```python
from build123d import *

# Parameters (mm, degrees)
MAIN_SIDE_DEPTH          = 3.175
SKETCH2_W                = 12.573
SKETCH2_H                = 3.048
BOTTOM_PLATE_HOLES_DEPTH = 254.555547868
SKETCH3_W                = 12.7
SKETCH3_H                = 3.048
CUT_EXTRUDE1_DEPTH       = 254.555547868
SKETCH4_W                = 3.048
SKETCH4_H                = 12.573
CUT_EXTRUDE2_DEPTH       = 254.555547868
SKETCH5_W                = 3.175
SKETCH5_H                = 31.75
CUT_EXTRUDE3_DEPTH       = 254.555547868
SKETCH6_R                = 9.525
CUT_EXTRUDE4_DEPTH       = 254.555547868
SKETCH7_W                = 12.7
SKETCH7_H                = 3.175
CUT_EXTRUDE5_DEPTH       = 254.555547868
SKETCH8_W                = 3.175
SKETCH8_H                = 12.7
CUT_EXTRUDE6_DEPTH       = 254.555547868
BOSS_EXTRUDE2_DEPTH      = 3.175
SKETCH10_R               = 1.75
SKETCH10_R_2             = 7.62
CUT_EXTRUDE7_DEPTH       = 254.555547868
FILLET1_R                = 6.35
SKETCH14_R               = 3.81
SKETCH14_W               = 3.175
SKETCH14_H               = 6.35
CUT_EXTRUDE8_DEPTH       = 254.555547868
CUT_EXTRUDE9_DEPTH       = 254.555547868
CUT_EXTRUDE10_DEPTH      = 254.555547868
FILLET2_R                = 6.35


with BuildPart() as part:
    # Sketch1 → Main Side (new body)
    with BuildSketch(Plane.XY):
        Polygon((62.123903317, 7.421650144), (131.966346795, 7.421650144), (147.472889282, 13.771650144), (201.808790274, 13.771650144), (201.808790274, 77.271650144), (151.008790274, 77.271650144), (151.008790274, 153.471650144), (86.008898009, 153.471650144), (79.342261849, 77.271650144), (-42.539209726, 77.271650144), (-42.539209726, 13.771650144), (46.617360741, 13.771650144), align=None)
    extrude(amount=MAIN_SIDE_DEPTH)

    # Sketch2 → Bottom Plate Holes (cut, through all)
    with BuildSketch(Plane.XY.offset(3.175)):
        with Locations((141.483790274, 29.265650144)):
            Rectangle(SKETCH2_W, SKETCH2_H)
        with Locations((20.833790274, 29.265650144)):
            Rectangle(SKETCH2_W, SKETCH2_H)
    extrude(amount=-BOTTOM_PLATE_HOLES_DEPTH, mode=Mode.SUBTRACT)

    # Sketch3 → Cut-Extrude1 (cut, through all)
    with BuildSketch(Plane.XY.offset(3.175)):
        with Locations((119.258790274, 70.413650144)):
            Rectangle(SKETCH3_W, SKETCH3_H)
    extrude(amount=-CUT_EXTRUDE1_DEPTH, mode=Mode.SUBTRACT)

    # Sketch4 → Cut-Extrude2 (cut, through all)
    with BuildSketch(Plane.XY.offset(3.175)):
        with Locations((-41.015209726, 45.521650144)):
            Rectangle(SKETCH4_W, SKETCH4_H)
    extrude(amount=-CUT_EXTRUDE2_DEPTH, mode=Mode.SUBTRACT)

    # Sketch5 → Cut-Extrude3 (cut, through all)
    with BuildSketch(Plane.XY.offset(3.175)):
        with Locations((193.871290274, 61.396650144)):
            Rectangle(SKETCH5_W, SKETCH5_H)
    extrude(amount=-CUT_EXTRUDE3_DEPTH, mode=Mode.SUBTRACT)

    # Sketch6 → Cut-Extrude4 (cut, through all)
    with BuildSketch(Plane.XY.offset(3.175)):
        with Locations((-2.114209726, 51.856650144)):
            Circle(SKETCH6_R)
    extrude(amount=-CUT_EXTRUDE4_DEPTH, mode=Mode.SUBTRACT)

    # Sketch7 → Cut-Extrude5 (cut, through all)
    with BuildSketch(Plane.XY.offset(3.175)):
        with Locations((118.508844141, 151.884150144)):
            Rectangle(SKETCH7_W, SKETCH7_H)
    extrude(amount=-CUT_EXTRUDE5_DEPTH, mode=Mode.SUBTRACT)

    # Sketch8 → Cut-Extrude6 (cut, through all)
    with BuildSketch(Plane.XY.offset(3.175)):
        with Locations((149.421290274, 115.371650144)):
            Rectangle(SKETCH8_W, SKETCH8_H)
    extrude(amount=-CUT_EXTRUDE6_DEPTH, mode=Mode.SUBTRACT)

    # Sketch13 → Boss-Extrude2 (add)
    with BuildSketch(Plane.XY.offset(3.175)):
        Polygon((33.917360741, 13.771650144), (56.482594802, -1.468349856), (137.607655293, -1.468349856), (160.172889282, 13.771650144), (147.472889282, 13.771650144), (131.966346795, 7.421650144), (62.123903317, 7.421650144), (46.617360741, 13.771650144), align=None)
    extrude(amount=-BOSS_EXTRUDE2_DEPTH)

    # Sketch10 → Cut-Extrude7 (cut, through all)
    with BuildSketch(Plane.XY.offset(3.175)):
        with Locations((84.460790274, 3.141650144)):
            Circle(SKETCH10_R)
        with Locations((104.460790274, 10.641650144)):
            Circle(SKETCH10_R_2)
        with BuildLine():
            Line((86.210790274, 21.734048116), (86.210790274, 14.549252171))
            ThreePointArc((86.210790274, 14.549252171), (84.460790274, 12.799252171), (82.710790274, 14.549252171))
            Line((82.710790274, 14.549252171), (82.710790274, 21.734048116))
            ThreePointArc((82.710790274, 21.734048116), (84.460790274, 23.484048116), (86.210790274, 21.734048116))
        make_face()
    extrude(amount=-CUT_EXTRUDE7_DEPTH, mode=Mode.SUBTRACT)

    # Fillet1
    fillet1_edges = [part.edges().sort_by_distance(p)[0] for p in [
        (33.917360741, 13.771650144, 1.5875),
        (160.172889282, 13.771650144, 1.5875),
        (137.607655293, -1.468349856, 1.5875),
        (56.482594802, -1.468349856, 1.5875),
        (-42.539209726, 13.771650144, 1.5875),
        (-42.539209726, 77.271650144, 1.5875),
        (79.342261849, 77.271650144, 1.5875),
        (86.008898009, 153.471650144, 1.5875),
        (151.008790274, 153.471650144, 1.5875),
        (201.808790274, 77.271650144, 1.5875),
        (201.808790274, 13.771650144, 1.5875),
    ]]
    fillet(fillet1_edges, radius=FILLET1_R - 0.0001)  # a hair under: the kernel refuses the full size

    # Sketch14 → Cut-Extrude8 (cut, through all)
    with BuildSketch(Plane.XY.offset(3.175)):
        with Locations((62.390480298, 6.151650144)):
            Circle(SKETCH14_R)
        with Locations((62.390480298, 72.191650144)):
            Circle(SKETCH14_R)
        with Locations((56.992980298, 63.936650144)):
            Rectangle(SKETCH14_W, SKETCH14_H)
        with Locations((67.787980298, 63.936650144)):
            Rectangle(SKETCH14_W, SKETCH14_H)
        with Locations((67.787980298, 14.406650144)):
            Rectangle(SKETCH14_W, SKETCH14_H)
        with Locations((56.992980298, 14.406650144)):
            Rectangle(SKETCH14_W, SKETCH14_H)
    extrude(amount=-CUT_EXTRUDE8_DEPTH, mode=Mode.SUBTRACT)

    # Sketch15 → Cut-Extrude9 (cut, through all)
    with BuildSketch(Plane.XY.offset(3.175)):
        Polygon((90.585226868, 85.563055457), (95.498090229, 141.717340628), (140.342125594, 141.717340628), (140.342125594, 85.563055457), align=None)
    extrude(amount=-CUT_EXTRUDE9_DEPTH, mode=Mode.SUBTRACT)

    # Sketch16 → Cut-Extrude10 (cut, through all)
    with BuildSketch(Plane.XY.offset(3.175)):
        Polygon((32.963134486, 23.931650144), (76.348530262, 23.931650144), (76.348530262, -1.468349856), (32.963134486, -1.468349856), (32.963134486, 12.534188724), (21.565673066, 12.534188724), align=None)
    extrude(amount=-CUT_EXTRUDE10_DEPTH, mode=Mode.SUBTRACT)

    # Fillet2
    fillet2_edges = [part.edges().sort_by_distance(p)[0] for p in [
        (22.803134486, 13.771650144, 1.5875),
        (76.348530262, -1.468349856, 1.5875),
        (32.963134486, 23.931650144, 1.5875),
        (76.348530262, 23.931650144, 1.5875),
    ]]
    fillet(fillet2_edges, radius=FILLET2_R)


solid = part.part
```
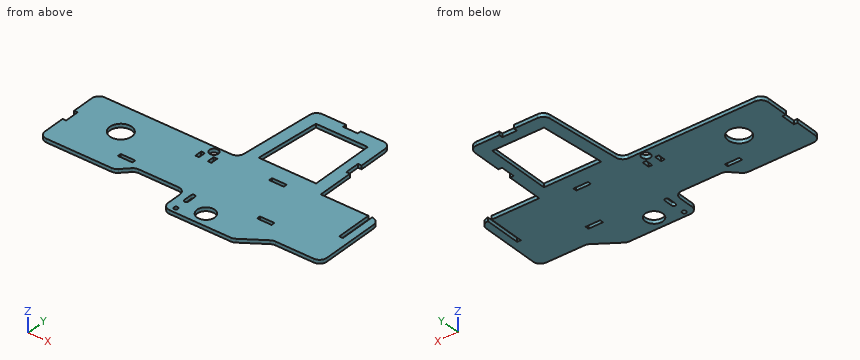
Could you check a few things on this model? Use its own coordinates, in mm. Round coordinates to 2 decimals unless told otherwise and drop trailing zeros. Write each loop counter-clockwise with the first axis right and the second up, starting at its lowest first coordinate (ties: lowest second). Pieces come first, ordered by that corner, then holes.
(1) Suppose I cut it at C-C on y = 125. Write out the boundary of the cut face in (x, z) (3 decimals).
Findings below:
outline: (83.518, 0) - (94.036, 0) - (94.036, 3.175) - (83.518, 3.175) - close; (140.342, 0) - (151.009, 0) - (151.009, 3.175) - (140.342, 3.175) - close
(2) For pin 1 (6 mm diameter, centred on x = 62.39, y = 72.19, fed in from +Z); pin 2 (0.9 mm diameter, centred on x = -41, z = 2, fed in from -Y); pin 3 (1 mm diameter, centred on x = 118.5, z = 1.5, fed in from +Y); pin 4 (1 mm diameter, centred on y = 87.5, z = 1.5, fed in from +X), each with a flat end and sliding along its axis, tell me the tip position at first contact or that it passes through.
Findings below:
pin 1: passes through
pin 2: stops at y = 15.51
pin 3: stops at y = 150.3
pin 4: stops at x = 151.01
(3) Suppose I cut it at D-D on z = 2.1. State how many separate pieces and enclosed holes the cut face has, and give its area (3 significant figures).
Findings below:
separate pieces: 1
enclosed holes: 11
area: 17,700 mm2
(4) If I drill on probe 1 along Y at (x, z) = (125, 0.35); probe 2 along X at (y, z) = (30, 2.4); probe 3 along X at (y, z) = (72, 1.7), over which ranges is the centre line in solid material (lowest first)?
Findings below:
probe 1: y = -1.47 to 68.89, 71.94 to 85.56, 141.72 to 153.47
probe 2: x = -42.54 to 14.55, 27.12 to 135.2, 147.77 to 201.81
probe 3: x = -42.45 to 58.59, 66.2 to 192.28, 195.46 to 201.72
(5) Suppose I cut it at B-B on y = 56. Write out the boundary of the cut face in (x, z) (3 decimals).
Findings below:
outline: (-42.539, 0) - (-10.691, 0) - (-10.691, 3.175) - (-42.539, 3.175) - close; (6.462, 0) - (192.284, 0) - (192.284, 3.175) - (6.462, 3.175) - close; (195.459, 0) - (201.809, 0) - (201.809, 3.175) - (195.459, 3.175) - close
(6) Suppose I cut it at A-A on x = 105.5. Write out the boundary of the cut face in (y, z) (3 decimals).
Findings below:
outline: (-1.468, 0) - (3.093, 0) - (3.093, 3.175) - (-1.468, 3.175) - close; (18.19, 0) - (85.563, 0) - (85.563, 3.175) - (18.19, 3.175) - close; (141.717, 0) - (153.472, 0) - (153.472, 3.175) - (141.717, 3.175) - close
